Input: dimensioned drawing with shaded views. Units: mm. Origin: part minimum x, y, z. Give positions to 0.01 mm unless a question says otherwise; leave off trailing zeros. Order: outer loops, then holes, each group sorted by start corner. A loop starts at its lowest first (then second) coordinate and runs counter-clockwise, first axis right, second up.
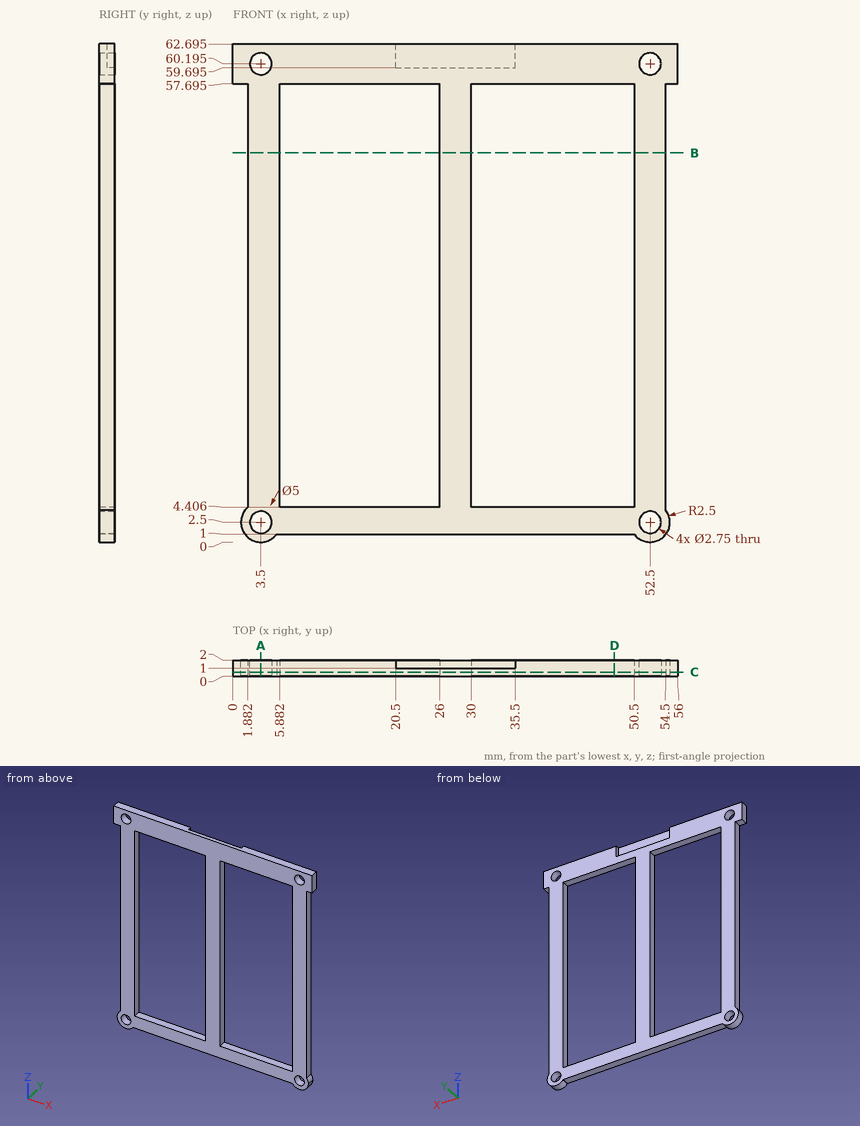
1) Cut plane D-D (x = 48). Return the cut outline in (y, z) (1 decimal), then the cut area to 3 significant figures.
2) Line query: probe 1 along X at (y, z) = (0.8, 45); probe 2 along X at (y, z) = (0.85, 2.5) (1 decimal); probe 3 along Z at (x, y) = (52.5, 1.25) (1 decimal). Output: solid intervals per line, ascending.
3) Cut plane A-A (x = 3.5). Return the cut outline in (y, z) (1 decimal).
4) First-contact query: P1, Ø4, axis at x = 28.5, z = 18.5, coming from the -Y side; P2, Ø2, axis at x = 3.5, z = 60.2, coming from the +Y side; P3, Ø0.6, axis at y = 1, z = 43, coming from the -X side; P4, Ø0.9, axis at x = 0.5, y = 0.5, coming from the -Z side (1 decimal). Flat tips, straight axial feed; report the tip coordinate or a pass-through.
5) Cut plane B-B (z = 49). Return the cut outline in (x, y), then the cut area to 3 significant figures.
6) Cut plane C-C (y = 0.5). Count the separate pieces of the cut face and the enclosed holes in it, then the cut area to 3 significant figures.
Geometry says:
1. outline: (0, 1) - (2, 1) - (2, 4.4) - (0, 4.4) - close; (0, 57.7) - (2, 57.7) - (2, 62.7) - (0, 62.7) - close
1. area: 16.8 mm2
2. probe 1: x = 1.88 to 5.88, 26 to 30, 50.5 to 54.5
2. probe 2: x = 1 to 2.1, 4.9 to 51.1, 53.9 to 55
2. probe 3: z = 0 to 1.1, 3.9 to 58.8, 61.6 to 62.7
3. outline: (0, 0) - (2, 0) - (2, 1.1) - (0, 1.1) - close; (0, 3.9) - (2, 3.9) - (2, 58.8) - (0, 58.8) - close; (0, 61.6) - (2, 61.6) - (2, 62.7) - (0, 62.7) - close
4. P1: stops at y = 0
4. P2: passes through
4. P3: stops at x = 1.88
4. P4: stops at z = 57.7
5. outline: (1.88, 0) - (5.88, 0) - (5.88, 2) - (1.88, 2) - close; (26, 0) - (30, 0) - (30, 2) - (26, 2) - close; (50.5, 0) - (54.5, 0) - (54.5, 2) - (50.5, 2) - close
5. area: 24.0 mm2
6. separate pieces: 1
6. enclosed holes: 6
6. area: 1,080 mm2
